Check sheet for the drawn part. Datum: minimum x, y, z corner. Units: mm. A direction names the side the tool comes from. Round coordinates to 2 decimals unless told otherwise and drop trailing zeros. Order: outer loops, then holes, each group sorted by start corner. A loop starts at its lowest first (then second) coordinate and runs counter-clockwise, first axis right, second up.
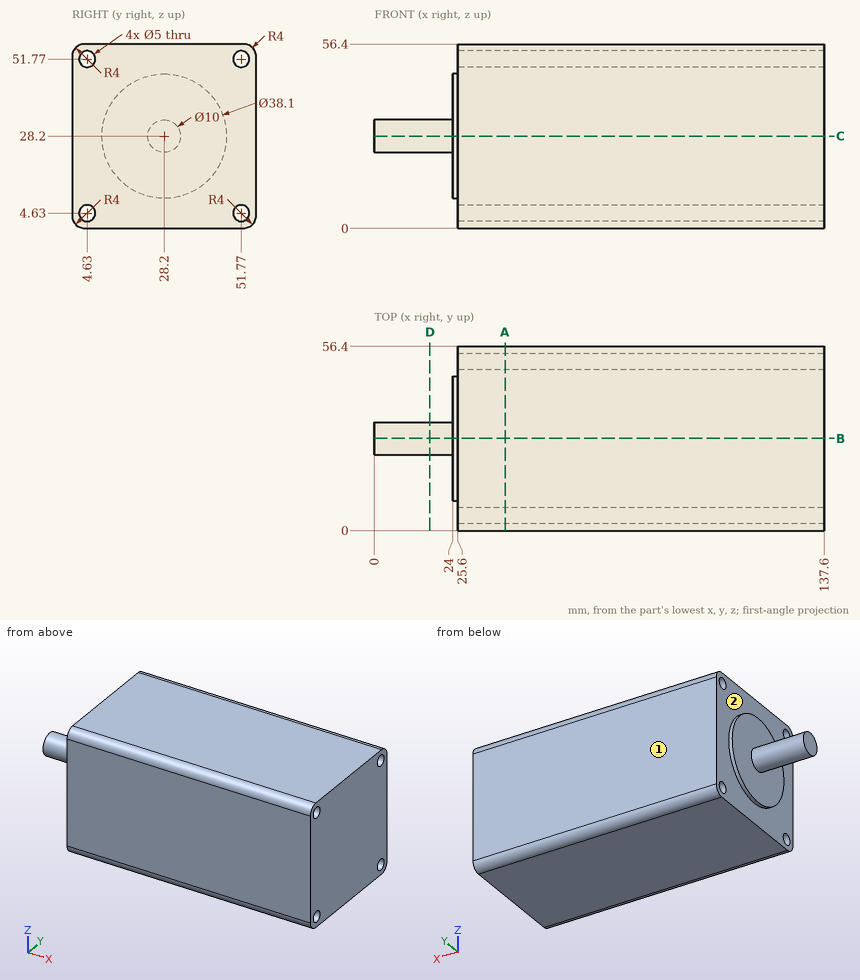
(1) Depth check by flat-ended pin: P1, Ø1, axis at y = 18, z = 38, coming from the -X side; P2, Ø5, axis at y = 32.5, z = 6.5, coming from the -X side. Enter the tip coordinate at first touch or a pass-through.
Returned:
P1: stops at x = 24
P2: stops at x = 25.6
(2) Set-up check for the marked faces 1 and 2: record each of +Z, -Z, +X, -X, +Y, -Y from which the full face is reachable in a straight line by a thin tool's end or side.
Returned:
face 1: +Z, -Z, +X, -X, +Y
face 2: -X
(3) Sectioned sample at D-D, the plane x = 17. Record the cut outline in (y, z), and give its area (3 significant figures).
Returned:
outline: circle Ø10 at (28.2, 28.2)
area: 78.5 mm2
(4) Sectioned sample at B-B, the plane y = 28.2. Record the cut outline in (x, z).
Returned:
outline: (0, 23.2) - (24, 23.2) - (24, 9.15) - (25.6, 9.15) - (25.6, 0) - (137.6, 0) - (137.6, 56.4) - (25.6, 56.4) - (25.6, 47.25) - (24, 47.25) - (24, 33.2) - (0, 33.2) - close
(5) Sectioned sample at A-A, the plane x = 40. Record the cut outline in (y, z).
Returned:
outline: (0, 4) arc R4 ccw to (4, 0) - (52.4, 0) arc R4 ccw to (56.4, 4) - (56.4, 52.4) arc R4 ccw to (52.4, 56.4) - (4, 56.4) arc R4 ccw to (0, 52.4) - close; hole circle Ø5 at (4.63, 4.63); hole circle Ø5 at (4.63, 51.77); hole circle Ø5 at (51.77, 4.63); hole circle Ø5 at (51.77, 51.77)
(6) Material ranges on line 1 (Y direction, x = 52, z = 51.77); line 2 (Y direction, x = 51, z = 4), recorded low to high.
Returned:
line 1: y = 0 to 2.13, 7.13 to 49.27, 54.27 to 56.4
line 2: y = 0 to 2.21, 7.05 to 49.35, 54.19 to 56.4
